The model under review builds one solid part; all positions refer to its coordinate system, in mm. Face numbers are marked on the shaded views. A direction names the side the tool comes from. Give positions to 0.01 mm unless a question says otherwise; leave off trailing zeros. Order: outer loops, then holes, each group sorted by start corner. A loop starts at its lowest first (then second) coordinate and runs counter-clockwise, first axis right, second up.
```python
from build123d import *

# Parameters (mm, degrees)
PAD012_DEPTH            = 39
HOLE003_D               = 5.8
HOLE003_DEPTH           = 50
HOLE003_CBORE_D         = 9.5
HOLE003_CBORE_DEPTH     = 5.4
HOLE003_TIPS_R          = 2.9
CHAMFER002_SIZE         = 1
SKETCH018_R             = 3.25
POCKET002_DEPTH         = 370.209154
BODY004_PLACEMENT_ANGLE = 270


with BuildPart() as part:
    # Sketch016 → Pad012 (new body, symmetric)
    with BuildSketch(Plane.XZ):
        with BuildLine():
            ThreePointArc((-32.484612, -1), (32.5, 0), (-32.484612, 1))
            Line((-49.5, 1), (-32.484612, 1))
            Line((-49.5, 1), (-49.5, 28))
            Line((-49.5, 28), (-37.749172, 28))
            ThreePointArc((37.749172, 28), (0, 47), (-37.749172, 28))
            Line((37.749172, 28), (49.5, 28))
            Line((49.5, 28), (49.5, -28))
            Line((64.5, -28), (49.5, -28))
            Line((64.5, -45), (64.5, -28))
            Line((-64.5, -45), (64.5, -45))
            Line((-64.5, -28), (-64.5, -45))
            Line((-49.5, -28), (-64.5, -28))
            Line((-49.5, -28), (-49.5, -1))
            Line((-32.484612, -1), (-49.5, -1))
        make_face()
    extrude(amount=PAD012_DEPTH, both=True)

    # Hole003
    with Locations(Plane(origin=(0, 0, 28), x_dir=(-1, 0, 0), z_dir=(0, 0, 1))):
        with Locations((43.624586, 0), (43.624586, 22.5), (43.624586, -22.5)):
            CounterBoreHole(HOLE003_D / 2, HOLE003_CBORE_D / 2, HOLE003_CBORE_DEPTH, depth=HOLE003_DEPTH)

    # Hole003 tips → Hole003 tip 1 section 0
    with BuildSketch(Plane(origin=(0, 0, -22), x_dir=(-1, 0, 0), z_dir=(0, 0, 1)), mode=Mode.PRIVATE) as hole003_tip_1_s0:
        with Locations((43.624586, 0)):
            Circle(HOLE003_TIPS_R)
    loft([hole003_tip_1_s0.sketch, Vertex(-43.624586, 0, -23.742496)], mode=Mode.SUBTRACT)

    # Hole003 tips → Hole003 tip 2 section 0
    with BuildSketch(Plane(origin=(0, 0, -22), x_dir=(-1, 0, 0), z_dir=(0, 0, 1)), mode=Mode.PRIVATE) as hole003_tip_2_s0:
        with Locations((43.624586, 22.5)):
            Circle(HOLE003_TIPS_R)
    loft([hole003_tip_2_s0.sketch, Vertex(-43.624586, -22.5, -23.742496)], mode=Mode.SUBTRACT)

    # Hole003 tips → Hole003 tip 3 section 0
    with BuildSketch(Plane(origin=(0, 0, -22), x_dir=(-1, 0, 0), z_dir=(0, 0, 1)), mode=Mode.PRIVATE) as hole003_tip_3_s0:
        with Locations((43.624586, -22.5)):
            Circle(HOLE003_TIPS_R)
    loft([hole003_tip_3_s0.sketch, Vertex(-43.624586, 22.5, -23.742496)], mode=Mode.SUBTRACT)

    # Chamfer002
    chamfer002_edges = [part.edges().sort_by_distance(p)[0] for p in [
        (32.5, 39, 0),
        (32.5, -39, 0),
        (0, -39, 47),
        (43.624586, -39, 28),
        (49.5, -39, 0),
        (57, -39, -28),
        (64.5, -39, -36.5),
        (-64.5, -39, -36.5),
        (-57, -39, -28),
        (-49.5, -39, -14.5),
        (-49.5, -39, 14.5),
        (0, -39, -45),
        (0, 39, 47),
        (-43.624586, 39, 28),
        (-49.5, 39, 14.5),
        (-49.5, 39, -14.5),
        (-57, 39, -28),
        (-64.5, 39, -36.5),
        (0, 39, -45),
        (64.5, 39, -36.5),
        (57, 39, -28),
        (49.5, 39, 0),
        (43.624586, 39, 28),
        (-64.5, 0, -45),
        (64.5, 0, -45),
    ]]
    chamfer(chamfer002_edges, length=CHAMFER002_SIZE)

    # Sketch018 (on Face51 of Chamfer002) → Pocket002 (cut, through all)
    with BuildSketch(Plane(origin=(0, 0, -28), x_dir=(-1, 0, 0), z_dir=(0, 0, 1))):
        with Locations((-57, 22.5)):
            Circle(SKETCH018_R)
        with Locations((-57, -22.5)):
            Circle(SKETCH018_R)
    pocket002 = extrude(amount=-POCKET002_DEPTH, mode=Mode.SUBTRACT)

    # Mirrored001: Pocket002 across YZ
    add(pocket002.mirror(Plane.YZ), mode=Mode.SUBTRACT)


with BuildPart() as part_1:
    # Body004 placement: moved
    add(part.part.moved(Location((-170, 173, 0))).rotate(Axis((-170, 173, 0), (1, 0, 0)), BODY004_PLACEMENT_ANGLE))


solid = part_1.part
```
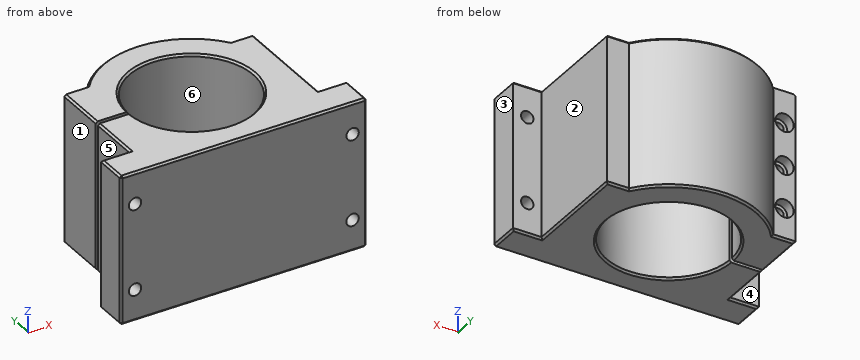
Item 1: Clearance check with flat-ended pins moving along their axes: pin 1 Ø8 at (y, z) = (192.5, 9.5) entering from -X; pin 2 Ø7.5 at (x, z) = (-227, 22.5) entering from +Y; pin 3 Ø5 at (y, z) = (201, 14.5) entering from +X; pin 4 Ø4 at (x, z) = (-113, -22.5) entering from +Y. State where each tip first meets the part, or that it passes through.
Values found:
pin 1: stops at x = -219.5
pin 2: stops at y = 145
pin 3: stops at x = -120.5
pin 4: passes through
Item 2: Take a section at B-B (x = -227). Give the boundary of the cut face in (y, z), and give its area (3 significant figures).
Values found:
outline: (128, -38) - (129, -39) - (144, -39) - (145, -38) - (145, -25.75) - (128, -25.75) - close; (128, -19.25) - (145, -19.25) - (145, 19.25) - (128, 19.25) - close; (128, 25.75) - (145, 25.75) - (145, 38) - (144, 39) - (129, 39) - (128, 38) - close
area: 1,100 mm2
Item 3: Take a section at D-D (x = -125). Give the boundary of the cut face in (y, z), and give its area (3 significant figures).
Values found:
outline: (128, -38) - (129, -39) - (200, -39) - (201, -38) - (201, 38) - (200, 39) - (129, 39) - (128, 38) - close
area: 5,690 mm2
Item 4: For line 1 (Z direction, x = -113, y = 141); line 2 (Y direction, x = -218, z = 17); line 3 (X direction, y = 156, z = 22), list the stretches that pass through material, from the lowest coordinate up.
Values found:
line 1: z = -39 to -25.75, -19.25 to 19.25, 25.75 to 39
line 2: y = 128 to 172, 174 to 201
line 3: x = -219.5 to -216.48, -210.77 to -197.7, -142.3 to -120.5
Item 5: Take a section at C-C (z = -31.5). Give the boundary of the cut face in (x, y), and give its area (3 significant figures).
Values found:
outline: (-234.5, 129) - (-233.5, 128) - (-106.5, 128) - (-105.5, 129) - (-105.5, 145) - (-120.5, 145) - (-120.5, 201) - (-132.25, 201) arc R47 ccw to (-207.75, 201) - (-219.5, 201) - (-219.5, 174) - (-202.48, 174) arc R32.5 cw (long way) to (-202.48, 172) - (-219.5, 172) - (-219.5, 145) - (-234.5, 145) - close
area: 5,390 mm2
Item 6: Draft analysis for pull direction Y (two halves, no side actions). For the marked faces 4, 5 and 6, state which applies: released by +Y, released by -Y, zero draft, split by the parting line, or undercut.
Values found:
face 4: released by +Y
face 5: zero draft
face 6: undercut
Item 7: Take a section at A-A (x = -170). Give the boundary of the cut face in (y, z), and give its area (3 significant figures).
Values found:
outline: (128, -38) - (129, -39) - (139.5, -39) - (140.5, -38) - (140.5, 38) - (139.5, 39) - (129, 39) - (128, 38) - close; (205.5, -38) - (206.5, -39) - (219, -39) - (220, -38) - (220, 38) - (219, 39) - (206.5, 39) - (205.5, 38) - close
area: 2,100 mm2
Item 8: For the marked faces 1, 2 and 3, list the 3-axis set-ups (+Z, -Z, +X, -X, +Y, -Y) from which the entire face can be reached by the end or side of a thin tool; tool diameter is ignored.
Values found:
face 1: +Z, -Z, -X, +Y
face 2: +Z, -Z, +X, +Y
face 3: +Z, -Z, +X, +Y, -Y
